```python
from build123d import *

# Parameters (mm, degrees)
SKETCH2_R           = 12.5
SKETCH2_R_2         = 2
BOSS_EXTRUDE2_DEPTH = 20
FILLET2_R           = 5


with BuildPart() as part:
    # Sketch2 → Boss-Extrude2 (new body)
    with BuildSketch(Plane(origin=(0, 0, 0), x_dir=(0, 0, -1), z_dir=(1, 0, 0))):
        Circle(SKETCH2_R)
        with BuildLine():
            Line((0, 3.5), (0, 7.5))
            ThreePointArc((0, 7.5), (1.463177415, 7.355889603), (2.870125743, 6.929096494))
            Line((2.870125743, 6.929096494), (1.339392013, 3.233578364))
            ThreePointArc((1.339392013, 3.233578364), (0.682816127, 3.432748481), (0, 3.5))
        make_face(mode=Mode.SUBTRACT)
        with BuildLine():
            Line((-2.870125743, 6.929096494), (-1.339392013, 3.233578364))
            ThreePointArc((-1.339392013, 3.233578364), (-1.944495816, 2.910143643), (-2.474873734, 2.474873734))
            Line((-2.474873734, 2.474873734), (-5.303300859, 5.303300859))
            ThreePointArc((-5.303300859, 5.303300859), (-4.166776748, 6.236022092), (-2.870125743, 6.929096494))
        make_face(mode=Mode.SUBTRACT)
        with BuildLine():
            Line((-6.929096494, 2.870125743), (-3.233578364, 1.339392013))
            ThreePointArc((-3.233578364, 1.339392013), (-3.432748481, 0.682816127), (-3.5, 0))
            Line((-3.5, 0), (-7.5, 0))
            ThreePointArc((-7.5, 0), (-7.355889603, 1.463177415), (-6.929096494, 2.870125743))
        make_face(mode=Mode.SUBTRACT)
        with BuildLine():
            Line((-6.929096494, -2.870125743), (-3.233578364, -1.339392013))
            ThreePointArc((-3.233578364, -1.339392013), (-2.910143643, -1.944495816), (-2.474873734, -2.474873734))
            Line((-2.474873734, -2.474873734), (-5.303300859, -5.303300859))
            ThreePointArc((-5.303300859, -5.303300859), (-6.236022092, -4.166776748), (-6.929096494, -2.870125743))
        make_face(mode=Mode.SUBTRACT)
        with BuildLine():
            Line((-2.870125743, -6.929096494), (-1.339392013, -3.233578364))
            ThreePointArc((-1.339392013, -3.233578364), (-0.682816127, -3.432748481), (0, -3.5))
            Line((0, -3.5), (0, -7.5))
            ThreePointArc((0, -7.5), (-1.463177415, -7.355889603), (-2.870125743, -6.929096494))
        make_face(mode=Mode.SUBTRACT)
        with BuildLine():
            Line((2.870125743, -6.929096494), (1.339392013, -3.233578364))
            ThreePointArc((1.339392013, -3.233578364), (1.944495816, -2.910143643), (2.474873734, -2.474873734))
            Line((2.474873734, -2.474873734), (5.303300859, -5.303300859))
            ThreePointArc((5.303300859, -5.303300859), (4.166776748, -6.236022092), (2.870125743, -6.929096494))
        make_face(mode=Mode.SUBTRACT)
        with BuildLine():
            Line((6.929096494, -2.870125743), (3.233578364, -1.339392013))
            ThreePointArc((3.233578364, -1.339392013), (3.432748481, -0.682816127), (3.5, 0))
            Line((3.5, 0), (7.5, 0))
            ThreePointArc((7.5, 0), (7.355889603, -1.463177415), (6.929096494, -2.870125743))
        make_face(mode=Mode.SUBTRACT)
        with BuildLine():
            Line((6.929096494, 2.870125743), (3.233578364, 1.339392013))
            ThreePointArc((3.233578364, 1.339392013), (2.910143643, 1.944495816), (2.474873734, 2.474873734))
            Line((2.474873734, 2.474873734), (5.303300859, 5.303300859))
            ThreePointArc((5.303300859, 5.303300859), (6.236022092, 4.166776748), (6.929096494, 2.870125743))
        make_face(mode=Mode.SUBTRACT)
        Circle(SKETCH2_R_2, mode=Mode.SUBTRACT)
    extrude(amount=BOSS_EXTRUDE2_DEPTH)

    # Fillet2
    fillet2_edges = [part.edges().sort_by_distance(p)[0] for p in [
        (0, 0, 12.5),
        (20, 0, 12.5),
    ]]
    fillet(fillet2_edges, radius=FILLET2_R - 0.0001)  # a hair under: the kernel refuses the full size


solid = part.part
```
The model under review builds one solid part; all positions refer to its coordinate system, in mm. A direction names the side the tool comes from. Round coordinates to 2 decimals unless told otherwise and drop trailing zeros. Write each question's results on one line, items separated by ' | '. Start each with the question number.
Q1. Insertion check: P1, Ø2, axis at x = 14.5, z = 7, coming from the +Y side; P2, Ø1.2, axis at x = 7.5, z = 4.5, coming from the +Y side; P3, Ø12, axis at y = 6, z = 3.5, coming from the +X side; P4, Ø2, axis at x = 13.5, z = -6, coming from the -Y side. Each pin has a flat end and moves straight along its axis. Give the tip position at first contact, or say it passes through.
Q2. Tool access review of faces 1 (the flat face through (0, 2, -2)), 2 (the flat face through (9.86, -5.107, 2.115)): name each direction out of +Z, -Z, +X, -X, +Y, -Y from which nothing blocks a thin tool from reaching the whole face with its end or side.
Q3. Wall thickness on line 1 along Y through (x, z) = (18, -1.5); line 2 along Z through (x, y) = (16.75, -6); line 3 along Z through (x, y) = (18, -6.75): over which ranges is each line inside the solid? List them lowest first. Write a range as [from, to].
Q4. Take a section at A-A on x = 8. Give the number of separate pieces and of enclosed holes in the cut face, plus the area to 3 significant figures.
Data:
1) P1: stops at y = 10.97 | P2: stops at y = 11.88 | P3: stops at x = 20 | P4: stops at y = -11.46
2) face 1: +Z, -Z, -X, +Y, -Y | face 2: +X, -X
3) line 1: y = [-11.4, -3.62], [-3.16, -1.32], [1.32, 3.62], [7.35, 11.4] | line 2: z = [-10.6, -4.5], [-2.49, 0], [2.49, 10.6] | line 3: z = [-9.31, -3.27], [-2.8, 0], [2.8, 9.31]
4) separate pieces: 1 | enclosed holes: 9 | area: 409 mm²
